Verification items for the finished model (mm, model axes). Coordinates: 2 decimals unless noted, no trailing zeros. Order: outer loops, then holes, each group sorted by start corner. A loop starts at its lowest first (then second) coordinate and runs counter-clockwise, first axis right, second up. Notation, with made-up numbers: M 73.25,66.25 L 132.25,66.25 A13 cw 132.25,83.25 Z; hole C 86.5,15 d7. An arc over 180 degrees is marked long. Answer as a JSON object with one key per item and string values. Group by question number.
(1) Material ranges on line 1 (X direction, y = -1.75, z = 0); line 2 (X direction, y = -10, z = -22); line 3 (Z direction, x = 22, y = 6.25), recorded low to high.
(2) Mould release check, pull along X, two halves, no side actions. Record for faces 1 (the face through (22, 12.7, 20)), 2 (the face through (-30.911, 0.124, -40.313)), 3 (the face through (-15.456, 0.124, -20.157)): released by +X, released by -X, zero draft, split by the parting line, or undercut.
(3) Gauge pin test, flat ends, axial feed: pin 1 Ø12 at (x, y) = (35, 2) entering from -Z; pin 2 Ø3 at (x, y) = (7, -0.5) entering from -Z; pin 3 Ø8 at (y, z) = (1.5, -38.5) entering from +X. Record the tip position at first contact, or that the pin passes through.
(4) Cross-section at C-C (y = -4.5). Enter the section's corners in (x, z), plus the area to 3 significant figures.
(5) Cross-section at A-A (x = 0). Enter the section's corners in (y, z).
(6) Cross-section at B-B (z = 0). Enter the section's corners in (x, y), plus the area to 3 significant figures.
from build123d import *

# Parameters (mm, degrees)
SKETCH2_R           = 50.8
BOSS_EXTRUDE3_DEPTH = 12.7
SKETCH4_R           = 25.4
CUT_EXTRUDE1_DEPTH  = 13.97
FILLET1_R           = 3.81
FILLET2_R           = 3.81
FILLET3_R           = 3.81
FILLET4_R           = 3.81


with BuildPart() as part:
    # Sketch2 → Boss-Extrude3 (new, symmetric)
    with BuildSketch(Plane(origin=(0, 0, 0), x_dir=(1, 0, 0), z_dir=(0, 1, 0))):
        with Locations(Location((0, 0, 0), (0, 0, 270))):
            Circle(SKETCH2_R)
    extrude(amount=BOSS_EXTRUDE3_DEPTH, both=True)

    # Sketch4 → Cut-Extrude1 (cut, symmetric)
    with BuildSketch(Plane(origin=(0, 0, 0), x_dir=(1, 0, 0), z_dir=(0, 1, 0))):
        with Locations(Location((0, 0, 0), (0, 0, 270))):
            Circle(SKETCH4_R)
    extrude(amount=CUT_EXTRUDE1_DEPTH, both=True, mode=Mode.SUBTRACT)

    # Fillet1
    fillet1_edges = [part.edges().sort_by_distance(p)[0] for p in [
        (0, -12.7, -50.8),
    ]]
    fillet(fillet1_edges, radius=FILLET1_R)

    # Fillet2
    fillet2_edges = [part.edges().sort_by_distance(p)[0] for p in [
        (0, -12.7, -25.4),
    ]]
    fillet(fillet2_edges, radius=FILLET2_R)

    # Fillet3
    fillet3_edges = [part.edges().sort_by_distance(p)[0] for p in [
        (0, 12.7, -50.8),
    ]]
    fillet(fillet3_edges, radius=FILLET3_R)

    # Fillet4
    fillet4_edges = [part.edges().sort_by_distance(p)[0] for p in [
        (0, 12.7, -25.4),
    ]]
    fillet(fillet4_edges, radius=FILLET4_R)


solid = part.part
Taken from the geometry:
{
 "1": {"line 1": "x = -50.8 to -25.4, 25.4 to 50.8", "line 2": "x = -45.61 to -13.02, 13.02 to 45.61", "line 3": "z = -45.79 to -12.69, 12.69 to 45.79"},
 "2": {"face 1": "zero draft", "face 2": "split by the parting line", "face 3": "undercut"},
 "3": {"pin 1": "stops at z = -41.71", "pin 2": "stops at z = -50.5", "pin 3": "stops at x = 37.29"},
 "4": {"outline": "C 0,0 d101.6; hole C 0,0 d50.8", "area": "6,080 mm²"},
 "5": {"outline": "M -12.7,-46.99 A3.81 ccw -8.89,-50.8 L 8.89,-50.8 A3.81 ccw 12.7,-46.99 L 12.7,-29.21 A3.81 ccw 8.89,-25.4 L -8.89,-25.4 A3.81 ccw -12.7,-29.21 Z; M -12.7,29.21 A3.81 ccw -8.89,25.4 L 8.89,25.4 A3.81 ccw 12.7,29.21 L 12.7,46.99 A3.81 ccw 8.89,50.8 L -8.89,50.8 A3.81 ccw -12.7,46.99 Z"},
 "6": {"outline": "M -50.8,-8.89 A3.81 ccw -46.99,-12.7 L -29.21,-12.7 A3.81 ccw -25.4,-8.89 L -25.4,8.89 A3.81 ccw -29.21,12.7 L -46.99,12.7 A3.81 ccw -50.8,8.89 Z; M 25.4,-8.89 A3.81 ccw 29.21,-12.7 L 46.99,-12.7 A3.81 ccw 50.8,-8.89 L 50.8,8.89 A3.81 ccw 46.99,12.7 L 29.21,12.7 A3.81 ccw 25.4,8.89 Z", "area": "1,270 mm²"}
}
